Input: part model. Units: mm. Frame: model coordinates. A direction names the side the tool comes from. Round coordinates to 2 decimals unless told otherwise and drop trailing zeros. Order: outer loops, then holes, each group sorted by start corner. A loop starts at its lowest first (then second) coordinate and runs counter-clockwise, first axis right, second up. Notation, with made-up numbers: M 11,31.5 L 24,31.5 A18 ccw 24,37.5 Z; hole C -16.5,-35.75 d4. An arc over 180 degrees is marked long. One line per question, with ' | ' between items.
```python
from build123d import *

# Parameters (mm, degrees)
F3_DEPTH     = 25.4
F5_DEPTH     = 2.54
F1_FACE_R    = 12.7
F6_DEPTH     = 0.6
F6_TAPER     = 45
F7_T4_ANGLE  = 71.9999997561
F7_T10_ANGLE = 72.000000061
F7_T16_ANGLE = 72.000000061
F7_T22_ANGLE = 72.000000061


# Not quite as in the source:
# - a fillet or chamfer that OpenCascade refuses, or shapes differently, is made with other operations: its cross-section is extruded or revolved along the edge and cut away or added


with BuildPart() as f1:
    # F0 (on Front) → F1 (revolve)
    with BuildSketch(Plane.XZ):
        Polygon((0, 10.656565316), (0, 0), (12.7, 0), align=None)
    revolve(axis=Axis((0, 0, 24.9413493462), (0, 0, 1)))

    # F2 (on Top) → F3 (join)
    with BuildSketch(Plane.XY):
        Polygon((-9.9684698397, 2.0625815326), (-8.5595086348, 2.7811529858), (-9.2770164791, 4.1906561266), (-11.0598678693, 4.7699396671), (-11.7513212299, 2.6418650731), align=None)
        Polygon((-1.1187950245, 10.1179509397), (0, 9), (1.1187950245, 10.1179509397), (1.1187950245, 11.9925518305), (-1.1187950245, 11.9925518305), align=None)
        Polygon((9.2770165014, 4.1906560772), (8.5595086496, 2.7811529403), (9.9684698507, 2.0625814795), (11.751321244, 2.6418650106), (11.0598678947, 4.7699396082), align=None)
        Polygon((6.8523065178, -7.5279830573), (5.2900672551, -7.2811529606), (5.0420581389, -8.8432054849), (6.1439208932, -10.3597894656), (7.9541692721, -9.044567038), align=None)
        Polygon((-5.0420581859, -8.8432054581), (-5.2900672939, -7.2811529325), (-6.8523065578, -7.5279830208), (-7.9541693202, -9.0445669956), (-6.1439209483, -10.3597894329), align=None)
    extrude(amount=F3_DEPTH)

    # F4 (on face) → F5 (join)
    with BuildSketch(Plane.XY.offset(25.4)):
        with BuildLine():
            ThreePointArc((-5.2900672939, -7.2811529325), (-4.0859144849, 8.0190587242), (9, 0))
            ThreePointArc((9, 0), (7.7919238303, -4.5039896783), (4.4920171062, -7.7988321124))
            Line((4.4920171062, -7.7988321124), (5.2905979251, -9.1852911546))
            ThreePointArc((5.2905979251, -9.1852911546), (9.1771547335, -5.3046989544), (10.6, 0))
            ThreePointArc((10.6, 0), (-4.306450321, 9.6857878168), (-7.1008463458, -7.8700686892))
            Line((-7.1008463458, -7.8700686892), (-6.8523065578, -7.5279830208))
            Line((-6.8523065578, -7.5279830208), (-5.2900672939, -7.2811529325))
        make_face()
        with BuildLine():
            ThreePointArc((-4.457782334, -7.8184510399), (-4.8813231204, -7.5612621033), (-5.2900672939, -7.2811529325))
            Line((-5.2900672939, -7.2811529325), (-5.0420581859, -8.8432054581))
            Line((-5.0420581859, -8.8432054581), (-4.457782334, -7.8184510399))
        make_face()
    extrude(amount=-F5_DEPTH)

    # F1_face (on face) → F6 (join)
    with BuildSketch(Plane(origin=(0, 0, 0), x_dir=(1, 0, 0), z_dir=(0, 0, -1))):
        Circle(F1_FACE_R)
    extrude(amount=F6_DEPTH, taper=F6_TAPER)

    # F7: chamfer of 1 on 4 edges, made by hand


with BuildPart() as f7_tool2:
    # F7_s3 → F7_t4 (revolve)
    with BuildSketch(Plane(origin=(0, 0, 0), x_dir=(0, 0, 1), z_dir=(-0.3090169984, -0.951056515, 0))):
        Polygon((22.86, 10), (23.86, 9), (22.86, 9), align=None)
    revolve(axis=Axis((0, 0, 22.86), (0, 0, -1)), revolution_arc=F7_T4_ANGLE)

    split(bisect_by=Plane(origin=(4.4999987183, 4.5033963456, 0), x_dir=(0, 0, 1), z_dir=(-0.7068398887, -0.707373573, 0)), keep=Keep.TOP)

    split(bisect_by=Plane(origin=(-5.6735605309, -2.888127077, 0), x_dir=(0, 0, 1), z_dir=(0.8911777859, 0.4536542229, 0)), keep=Keep.TOP)


with BuildPart() as f1_1:
    add(f1.part)

    # F7_t1: cut F7_tool2
    add(f7_tool2.part, mode=Mode.SUBTRACT)


with BuildPart() as f7_tool8:
    # F7_s9 → F7_t10 (revolve)
    with BuildSketch(Plane(origin=(0, 0, 0), x_dir=(0, 0, 1), z_dir=(0.8090169925, -0.5877852549, 0))):
        Polygon((22.86, 10), (23.86, 9), (22.86, 9), align=None)
    revolve(axis=Axis((0, 0, 22.86), (0, 0, -1)), revolution_arc=F7_T10_ANGLE)

    split(bisect_by=Plane(origin=(-2.8924083372, 5.6713791199, 0), x_dir=(0, 0, 1), z_dir=(0.4543267043, -0.8908351395, 0)), keep=Keep.TOP)

    split(bisect_by=Plane(origin=(0.9935454605, -6.2883570612, 0), x_dir=(0, 0, 1), z_dir=(-0.1560617251, 0.9877473047, 0)), keep=Keep.TOP)


with BuildPart() as f1_2:
    add(f1_1.part)

    # F7_t7: cut F7_tool8
    add(f7_tool8.part, mode=Mode.SUBTRACT)


with BuildPart() as f7_tool14:
    # F7_s15 → F7_t16 (revolve)
    with BuildSketch(Plane.YZ):
        Polygon((10, 22.86), (9, 23.86), (9, 22.86), align=None)
    revolve(axis=Axis((0, 0, 22.86), (0, 0, -1)), revolution_arc=F7_T16_ANGLE)

    split(bisect_by=Plane(origin=(5.6735605155, -2.8881271072, 0), x_dir=(0, 0, 1), z_dir=(-0.8911777835, 0.4536542277, 0)), keep=Keep.TOP)

    split(bisect_by=Plane(origin=(-4.4999987183, 4.5033963456, 0), x_dir=(0, 0, 1), z_dir=(0.7068398887, -0.707373573, 0)), keep=Keep.TOP)


with BuildPart() as f1_3:
    add(f1_2.part)

    # F7_t13: cut F7_tool14
    add(f7_tool14.part, mode=Mode.SUBTRACT)


with BuildPart() as f7_tool20:
    # F7_s21 → F7_t22 (revolve)
    with BuildSketch(Plane(origin=(0, 0, 0), x_dir=(0, 0, 1), z_dir=(-0.3090169934, 0.9510565166, 0))):
        Polygon((22.86, 10), (23.86, 9), (22.86, 9), align=None)
    revolve(axis=Axis((0, 0, 22.86), (0, 0, -1)), revolution_arc=F7_T22_ANGLE)

    split(bisect_by=Plane(origin=(2.8924083674, 5.6713791045, 0), x_dir=(0, 0, 1), z_dir=(-0.4543267091, -0.8908351371, 0)), keep=Keep.TOP)

    split(bisect_by=Plane(origin=(-0.993545494, -6.2883570559, 0), x_dir=(0, 0, 1), z_dir=(0.1560617303, 0.9877473039, 0)), keep=Keep.TOP)


with BuildPart() as f1_4:
    add(f1_3.part)

    # F7_t19: cut F7_tool20
    add(f7_tool20.part, mode=Mode.SUBTRACT)


solid = f1_4.part
```
Item 1: Section query A-A, the plane z = 17.5. Return loops of the section in (x, y).
Report:
outline: M -11.75,2.64 L -9.97,2.06 L -8.56,2.78 L -9.28,4.19 L -11.06,4.77 Z; M -7.95,-9.04 L -6.14,-10.36 L -5.04,-8.84 L -5.29,-7.28 L -6.85,-7.53 Z; M -1.12,10.12 L 0,9 L 1.12,10.12 L 1.12,11.99 L -1.12,11.99 Z; M 5.04,-8.84 L 6.14,-10.36 L 7.95,-9.04 L 6.85,-7.53 L 5.29,-7.28 Z; M 8.56,2.78 L 9.97,2.06 L 11.75,2.64 L 11.06,4.77 L 9.28,4.19 Z
Item 2: Section query C-C, the plane z = 1.75. Return loops of the section in (x, y).
Report:
outline: M -11.75,2.64 L -10.38,2.2 A10.61 ccw -7.11,-7.88 L -7.95,-9.04 L -6.14,-10.36 L -5.3,-9.2 A10.61 ccw 5.3,-9.2 L 6.14,-10.36 L 7.95,-9.04 L 7.11,-7.88 A10.61 ccw 10.38,2.2 L 11.75,2.64 L 11.06,4.77 L 9.69,4.33 A10.61 ccw 1.12,10.56 L 1.12,11.99 L -1.12,11.99 L -1.12,10.56 A10.61 ccw -9.69,4.33 L -11.06,4.77 Z
Item 3: Section query D-D, the plane y = -4.25. Give the number of separate pieces and of enclosed holes in the cut face, plus the area to 3 significant figures.
Report:
separate pieces: 3 | enclosed holes: 0 | area: 123 mm²
Item 4: Mould query, pull axis X, two halves, no side actions, for faces 6 (the flat face through (-11.4, 3.72, 12.8)), 7 (the flat face through (-0.05, 9.15, 25.4)), 8 (the flat face through (4.77, -8.28, 24.15)). Classes: +X half, -X half, draft (parallel to the pull), parting line (faces both ways), or undercut.
Report:
face 6: -X half | face 7: draft | face 8: undercut
Item 5: First-contact query: pin 1 (1.5 mm diameter, centred on y = 11.5, z = 15.5, fed in from +X); pin 2 (5 mm diameter, centred on y = -10, z = 21.5, fed in from -X); pin 3 (8 mm diameter, centred on y = 7.5, z = 16.5, fed in from -X); pin 4 (5 mm diameter, centred on x = 10, y = 7, fed in from +Z). Flat tips, straight axial feed; report the tip coordinate or a pass-through.
Report:
pin 1: x = 1.12 | pin 2: x = -7.95 | pin 3: x = -11.47 | pin 4: z = 25.4
Item 6: Access query for faces 1 (the conical face through (-2.73, -2.09, 7.77)), 2 (the flat face through (-7.062, -9.693, 12.801)), 3 (the flat face through (10.181, 4.484, 12.801)), 4 (the flat face through (-7.4, -8.28, 12.8)), 5 (the flat face through (5.585, -9.591, 12.801)). Directions: +Z, -Z, +X, -X, +Y, -Y. A direction counts if a zero-diameter tool reaches every point of the face in a straight line with its end or side. Return the directions, or none.
Report:
face 1: none | face 2: +Z, -X, -Y | face 3: +Y | face 4: -X | face 5: +Z, -Y
Item 7: Line query: line 1 along X through (y, z) = (0, 24.65); line 2 along X through (y, z) = (-8, 22.5); line 3 along Y through (x, z) = (0, 24.6). Output: solid intervals per line, ascending. Write a range as from..to.
Report:
line 1: -10.6..-9, 9..10.6 | line 2: -7.2..-5.18, 5.18..7.2 | line 3: 9..11.99
Item 8: Section query B-B, the plane z = 4.5. Return loops of the section in (x, y), plus the area to 3 significant figures.
Report:
outline: M -11.75,2.64 L -9.97,2.06 L -8.56,2.78 L -9.28,4.19 L -11.06,4.77 Z; M -7.95,-9.04 L -6.14,-10.36 L -5.04,-8.84 L -5.29,-7.28 L -6.85,-7.53 Z; C 0,0 d14.67; M -1.12,10.12 L 0,9 L 1.12,10.12 L 1.12,11.99 L -1.12,11.99 Z; M 5.04,-8.84 L 6.14,-10.36 L 7.95,-9.04 L 6.85,-7.53 L 5.29,-7.28 Z; M 8.56,2.78 L 9.97,2.06 L 11.75,2.64 L 11.06,4.77 L 9.28,4.19 Z | area: 196 mm²
